CAD build for the part. Positions are in the model's coordinates, mm. A direction names the side the tool comes from. Give positions to 0.01 mm unless a question says otherwise; leave off trailing zeros. Loops run counter-clockwise (first coordinate to the right, second up) from the corner with the lowest first, then second, coordinate; pieces in that order, holes last.
```python
from build123d import *

# Parameters (mm, degrees)
SKETCH1_R           = 5
BOSS_EXTRUDE1_DEPTH = 9
BOSS_EXTRUDE2_DEPTH = 7.5
SKETCH3_R           = 5.5
BOSS_EXTRUDE3_DEPTH = 4
BOSS_EXTRUDE3_TAPER = 13
SKETCH4_R           = 5.6
BOSS_EXTRUDE4_DEPTH = 2
SKETCH5_R           = 3.175
CUT_EXTRUDE1_DEPTH  = 13
SKETCH6_R           = 2
CUT_EXTRUDE2_DEPTH  = 25.295061227
CHAMFER1_SIZE       = 1
CHAMFER2_SIZE       = 0.5


with BuildPart() as part:
    # Sketch1 → Boss-Extrude1 (new body)
    with BuildSketch(Plane.XY):
        Circle(SKETCH1_R)
    extrude(amount=BOSS_EXTRUDE1_DEPTH)

    # Sketch2 → Boss-Extrude2 (add)
    with BuildSketch(Plane.XY.offset(9)):
        Polygon((6.92820323, 0), (3.464101615, 6), (-3.464101615, 6), (-6.92820323, 0), (-3.464101615, -6), (3.464101615, -6), align=None)
    extrude(amount=BOSS_EXTRUDE2_DEPTH)

    # Sketch3 → Boss-Extrude3 (add)
    with BuildSketch(Plane.XY.offset(16.5)):
        Circle(SKETCH3_R)
    extrude(amount=BOSS_EXTRUDE3_DEPTH, taper=BOSS_EXTRUDE3_TAPER)

    # Sketch4 → Boss-Extrude4 (add)
    with BuildSketch(Plane.XY.offset(20.5)):
        Circle(SKETCH4_R)
    extrude(amount=BOSS_EXTRUDE4_DEPTH)

    # Sketch5 → Cut-Extrude1 (cut)
    with BuildSketch(Plane.XY.offset(22.5)):
        Circle(SKETCH5_R)
    extrude(amount=-CUT_EXTRUDE1_DEPTH, mode=Mode.SUBTRACT)

    # Sketch6 → Cut-Extrude2 (cut, through all)
    with BuildSketch(Plane(origin=(0, 0, 0), x_dir=(-1, 0, 0), z_dir=(0, 0, -1))):
        Circle(SKETCH6_R)
    extrude(amount=-CUT_EXTRUDE2_DEPTH, mode=Mode.SUBTRACT)

    # Sketch7 → Cut-Revolve1 (revolve, cut)
    with BuildSketch(Plane(origin=(0, 0, 0), x_dir=(1, 0, 0), z_dir=(0, 1, 0)), mode=Mode.PRIVATE) as cut_revolve1_sk:
        Polygon((5, -9), (6.92820323, -10), (6.92820323, -9), align=None)
        Polygon((6.92820323, -15.5), (6.92820323, -16.5), (5.5, -16.5), align=None)
    revolve(cut_revolve1_sk.sketch.rotate(Axis((0, 0, -1.125), (0, 0, 1)), 180), axis=Axis((0, 0, -1.125), (0, 0, 1)), mode=Mode.SUBTRACT)

    # Chamfer1
    chamfer1_edges = [part.edges().sort_by_distance(p)[0] for p in [
        (-5, 0, 0),
    ]]
    chamfer(chamfer1_edges, length=CHAMFER1_SIZE)

    # Chamfer2
    chamfer2_edges = [part.edges().sort_by_distance(p)[0] for p in [
        (2, 0, 0),
    ]]
    chamfer(chamfer2_edges, length=CHAMFER2_SIZE)


solid = part.part
```
1. Saw through at B-B, the plane x = 0. List the corners of the cut face in (y, z) (3 decimals), and give its area (3 significant figures).
Responses:
outline: (-6, 9.519) - (-5, 9) - (-5, 1) - (-4, 0) - (-2.5, 0) - (-2, 0.5) - (-2, 9.5) - (-3.175, 9.5) - (-3.175, 22.5) - (-5.6, 22.5) - (-5.6, 20.5) - (-4.577, 20.5) - (-5.5, 16.5) - (-6, 16.15) - close; (2, 0.5) - (2.5, 0) - (4, 0) - (5, 1) - (5, 9) - (6, 9.519) - (6, 16.15) - (5.5, 16.5) - (4.577, 20.5) - (5.6, 20.5) - (5.6, 22.5) - (3.175, 22.5) - (3.175, 9.5) - (2, 9.5) - close
area: 120 mm2
2. Saw through at A-A, the plane z = 14.5. List the corners of the cut face in (x, y) (3 decimals).
Responses:
outline: (-6.928, 0) - (-3.464, -6) - (3.464, -6) - (6.928, 0) - (3.464, 6) - (-3.464, 6) - close; hole circle Ø6.35 at (0, 0)
3. Tool access for faces 4 (the face through (-5.22, -2.96, 12.79)), 5 (the face through (-5.595, 0.246, 21.486)), 6 (the face through (4.604, 1.45, 19.417)): list every direction of +Z, -Z, +X, -X, +Y, -Y with a clear straight run to the whole face (end or side of a thin tool).
Responses:
face 4: +Z, -Z, -X, -Y
face 5: +Z
face 6: none
4. Drop flat-ended pins along their axis: pin 1 (3.5 mm diameter, centred on x = 0.5, y = -2.5, fed in from -Z); pin 2 (2 mm diameter, centred on y = 2.5, z = 6.5, fed in from +X); pin 3 (3 mm diameter, centred on y = -1, z = 7, fed in from +X). Give the stop position or say it passes through.
Responses:
pin 1: stops at z = 0
pin 2: stops at x = 4.77
pin 3: stops at x = 5
5. Probe line 1 along Y through (x, z) = (0, 12.75) (3 decimals); line 2 along Y through (x, z) = (0, 2.5); line 3 along X through (y, z) = (-0.25, 14). List the from-to ranges inside material, lowest first.
Responses:
line 1: y = -6 to -3.175, 3.175 to 6
line 2: y = -5 to -2, 2 to 5
line 3: x = -6.78 to -3.17, 3.17 to 6.78
6. Saw through at D-D, the plane z = 17.25. List the corners of the cut face in (x, y) (3 decimals), and give its area (3 significant figures).
Responses:
outline: circle Ø10.654 at (0, 0); hole circle Ø6.35 at (0, 0)
area: 57.5 mm2
7. Pull direction X, two halves, no side cores. Call faces 1 (the face through (-1.08, -4.88, 4.94)), 2 (the face through (1, -2, 9.5)), 3 (the face through (-5, 0, 20.5)): released by +X, released by -X, zero draft, split by the parting line, or undercut.
Responses:
face 1: split by the parting line
face 2: undercut
face 3: zero draft
8. Saw through at C-C, the plane z = 5. List the corners of the cut face in (x, y).
Responses:
outline: circle Ø10 at (0, 0); hole circle Ø4 at (0, 0)
